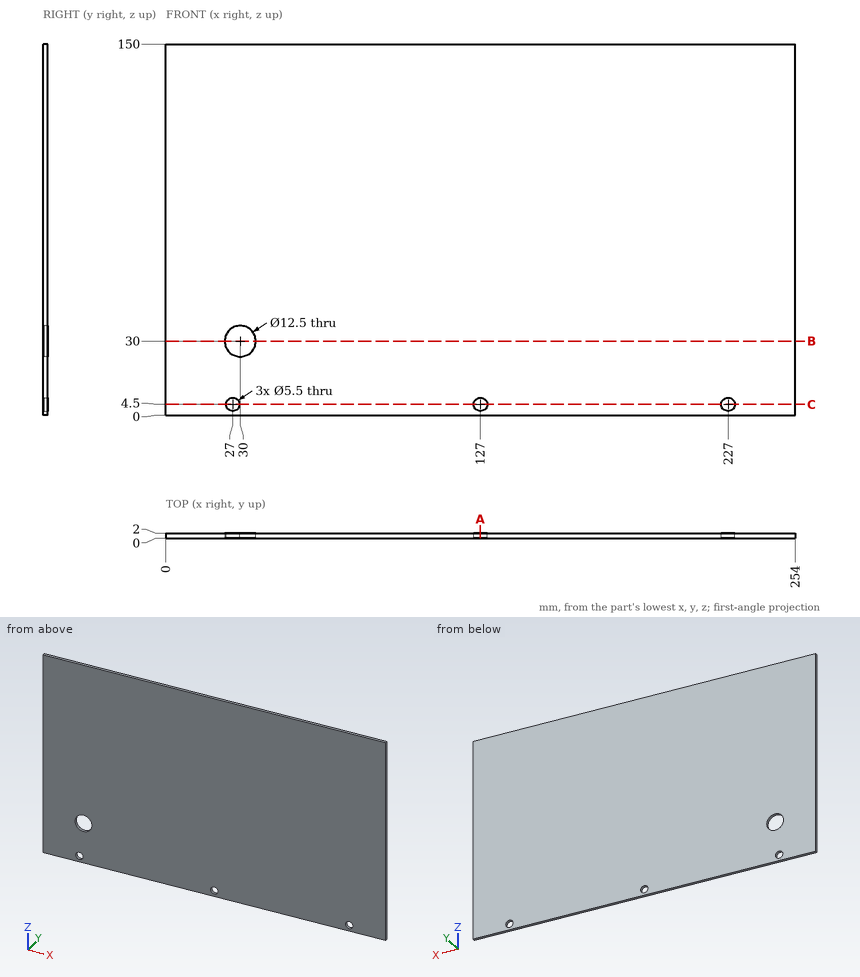
Geometry check sheet. Reference: drawing and pictorial views, mm from the part's lowest x, y, z. Round coordinates to 2 decimals unless told otherwise and drop trailing zeros. Loops run counter-clockwise (first coordinate to the right, second up) from the corner with the lowest first, then second, coordinate; pieces in that order, holes last.
1. Sectioned sample at A-A on x = 127. Record the boundary of the cut face in (y, z).
2. Scan lines: probe 1 along Z at (x, y) = (127, 1.25); probe 2 along Z at (x, y) = (30, 0.85); probe 3 along Z at (x, y) = (27, 0.8). Record each from-to range of solid material in increasing order.
3. Sectioned sample at B-B on z = 30. Record the boundary of the cut face in (x, y), and give its area (3 significant figures).
4. Sectioned sample at C-C on z = 4.5. Record the boundary of the cut face in (x, y).
Recorded:
1. outline: (0, 0) - (2, 0) - (2, 1.75) - (0, 1.75) - close; (0, 7.25) - (2, 7.25) - (2, 150) - (0, 150) - close
2. probe 1: z = 0 to 1.75, 7.25 to 150
2. probe 2: z = 0 to 23.75, 36.25 to 150
2. probe 3: z = 0 to 1.75, 7.25 to 24.52, 35.48 to 150
3. outline: (0, 0) - (23.75, 0) - (23.75, 2) - (0, 2) - close; (36.25, 0) - (254, 0) - (254, 2) - (36.25, 2) - close
3. area: 483 mm2
4. outline: (0, 0) - (24.25, 0) - (24.25, 2) - (0, 2) - close; (29.75, 0) - (124.25, 0) - (124.25, 2) - (29.75, 2) - close; (129.75, 0) - (224.25, 0) - (224.25, 2) - (129.75, 2) - close; (229.75, 0) - (254, 0) - (254, 2) - (229.75, 2) - close
